Autodesk Fusion 360 part; units mm, degrees
sketch "Sketch1" plane through (0, 0, 0) normal (0, 0, 1) x (1, 0, 0)
  circle A0 centre (0, 0) radius 20
  dimension "d1" = 40
extrude "Extrude1" add sketch "Sketch1" along normal blind 2
sketch "Sketch2" plane through (0, 0, 2) normal (0, 0, 1) x (-1, 0, 0)
  circle A0 centre (0, 0) radius 20
  line L0 (10, -10) -> (-10, -10) construction
  line L1 (-10, -10) -> (-10, 10) construction
  line L2 (-10, 10) -> (10, 10) construction
  line L3 (10, 10) -> (10, -10) construction
  circle A1 centre (10, -10) radius 1.5
  circle A2 centre (-10, -10) radius 1.5
  circle A3 centre (10, 10) radius 1.5
  circle A4 centre (-10, 10) radius 1.5
  dimension "d4" = 10
  dimension "d5" = 10
  dimension "d6" = 3
  dimension "d7" = 3
  dimension "d8" = 3
  dimension "d9" = 3
hole "Hole1" at (-10, -10, 2) at (-10, 10, 2) at (10, 10, 2) at (10, -10, 2) direction (0, 0, -1) diameter 2.529 depth 2 tip angle 118
Model file for the job. Use its own axes, mm. Round coordinates to 2 decimals unless told otherwise and drop trailing zeros. Order: outer loops, then holes, each group sorted by start corner. A loop starts at its lowest first (then second) coordinate and runs counter-clockwise, first axis right, second up.
(1) Pull direction Y, two halves, no side cores. Call faces 1 (the face through (-4.336, 19.524, 0.986)), 2 (the face through (0, 0, 2)), 3 (the face through (-9.231, 11.003, 0.986)): released by +Y, released by -Y, zero draft, split by the parting line, or undercut.
(2) Band-saw the part on B-B (z = 1.05). List the corners of the cut face in (x, y).
(3) Band-saw the part on A-A (y = 10). List the corners of the cut face in (x, z).
(4) Drill centre lines: line 1 (Y direction, x = -10.5, z = 0.1); line 2 (X direction, y = 10, z = 0.5); line 3 (Y direction, x = -11, z = 1.2). Where is each one in solid material? Low to high.
(5) Band-saw the part on D-D (x = 5). List the corners of the cut face in (y, z), then the cut area to 3 significant figures.
(6) Pin check, flat tips, straight feed: pin 1 (4 mm diameter, centred on x = -10, y = -10, fed in from +Z); pin 2 (1 mm diameter, centred on x = 12, z = 1, fed in from +Y). Stop position of each tip, or through.
Verdict:
1. face 1: split by the parting line
1. face 2: zero draft
1. face 3: undercut
2. outline: circle Ø40 at (0, 0); hole circle Ø2.53 at (-10, -10); hole circle Ø2.53 at (-10, 10); hole circle Ø2.53 at (10, -10); hole circle Ø2.53 at (10, 10)
3. outline: (-17.32, 0) - (-11.26, 0) - (-11.26, 2) - (-17.32, 2) - close; (-8.74, 0) - (8.74, 0) - (8.74, 2) - (-8.74, 2) - close; (11.26, 0) - (17.32, 0) - (17.32, 2) - (11.26, 2) - close
4. line 1: y = -17.02 to -11.16, -8.84 to 8.84, 11.16 to 17.02
4. line 2: x = -17.32 to -11.26, -8.74 to 8.74, 11.26 to 17.32
4. line 3: y = -16.7 to -10.77, -9.23 to 9.23, 10.77 to 16.7
5. outline: (-19.36, 0) - (19.36, 0) - (19.36, 2) - (-19.36, 2) - close
5. area: 77.5 mm2
6. pin 1: stops at z = 2
6. pin 2: stops at y = 16.36
